Here's how the part is built. I have some questions about the finished solid (model axes, mm). A direction names the side the tool comes from. Give positions to 0.01 mm unless a question says otherwise; leave off trailing zeros. Write each loop counter-clockwise with the first axis right and the second up, starting at its lowest first coordinate (ties: lowest second). Pieces come first, ordered by that corner, then holes. Notation, with made-up numbers: (47, -31) - (54, -31) arc R22 cw to (54, -6) - close; hole circle Ø3 at (42.5, 2.5). An arc over 180 degrees is marked (long way). Use a Markdown table: item, result.
```python
from build123d import *

# Parameters (mm, degrees)
BOSS_EXTRUDE1_DEPTH      = 25.4
BOSS_EXTRUDE1_DEPTH_BACK = 25.4
SKETCH3_R                = 8.382
CUT_EXTRUDE9_DEPTH       = 95.36535858
CUT_EXTRUDE14_DEPTH      = 63.5
SKETCH14_W               = 38.1
SKETCH14_H               = 46.622003784
CUT_EXTRUDE23_DEPTH      = 12.7
CUT_EXTRUDE23_DRAFT      = -8
SKETCH13_W               = 5.08
SKETCH13_H               = 2.54
CUT_EXTRUDE22_DEPTH      = 105.116765701
FILLET4_R                = 25.4
CUT_EXTRUDE24_REACH      = 96.365
SKETCH17_R               = 7.62
SKETCH17_R_2             = 2.032
CUT_EXTRUDE25_DEPTH      = 95.36535858
FILLET5_R                = 1.27
SKETCH17_7_R             = 2.032
CUT_EXTRUDE26_DEPTH      = 12.7
SKETCH18_R               = 7.62
CUT_EXTRUDE27_DEPTH      = 12.7


with BuildPart() as part:
    # Sketch1 → Boss-Extrude1 (new, two sides: drawn at the far end of the back side and taken through both)
    with BuildSketch(Plane(origin=(0, 0, 0), x_dir=(0, 0, -1), z_dir=(1, 0, 0)).offset(-BOSS_EXTRUDE1_DEPTH_BACK)):
        Polygon((0, 0), (6.960987543, 49.53), (76.2, 49.53), (76.2, 0), align=None)
    extrude(amount=BOSS_EXTRUDE1_DEPTH + BOSS_EXTRUDE1_DEPTH_BACK)

    # Sketch3 → Cut-Extrude9 (cut, through all)
    with BuildSketch(Plane.XZ):
        with Locations(Location((0, -63.246, 0), (0, 0, 270))):
            Circle(SKETCH3_R)
        with Locations(Location((0, -25.4, 0), (0, 0, 270))):
            Circle(SKETCH3_R)
    extrude(amount=-CUT_EXTRUDE9_DEPTH, mode=Mode.SUBTRACT)

    # Sketch9 → Cut-Extrude14 (cut)
    with BuildSketch(Plane(origin=(0, 0, -76.2), x_dir=(-1, 0, 0), z_dir=(0, 0, -1))):
        Polygon((-15.24, 49.53), (-15.24, 29.21), (-11.43, 29.21), (-11.43, 25.4), (-19.05, 25.4), (-19.05, 0), (19.05, 0), (19.05, 25.4), (11.43, 25.4), (11.43, 29.21), (15.24, 29.21), (15.24, 49.53), align=None)
    extrude(amount=-CUT_EXTRUDE14_DEPTH, mode=Mode.SUBTRACT)


with BuildPart() as cut_extrude23_tool:
    # Sketch14 → Cut-Extrude23 (with draft: the straight prism first)
    with BuildSketch(Plane.XZ):
        with Locations((0, -29.661001892)):
            Rectangle(SKETCH14_W, SKETCH14_H)
    extrude(amount=-CUT_EXTRUDE23_DEPTH)
    # Cut-Extrude23: the draft: its side faces are tilted about the plane it starts from
    cut_extrude23_sides = [cut_extrude23_tool.faces().sort_by_distance(p)[0] for p in [
        (0, 6.35, -6.35),
        (-19.05, 6.35, -29.661001892),
        (0, 6.35, -52.972003784),
        (19.05, 6.35, -29.661001892),
    ]]
    draft(cut_extrude23_sides, Plane.XZ, CUT_EXTRUDE23_DRAFT)


with BuildPart() as part_1:
    add(part.part)

    # Cut-Extrude23: cut by cut_extrude23_tool
    add(cut_extrude23_tool.part, mode=Mode.SUBTRACT)

    # Sketch13 → Cut-Extrude22 (cut, through all)
    with BuildSketch(Plane.ZY.offset(25.4)):
        with Locations((-70.485, 25.4)):
            Rectangle(SKETCH13_W, SKETCH13_H)
        with Locations((-34.900987543, 25.4)):
            Rectangle(SKETCH13_W, SKETCH13_H)
    extrude(amount=-CUT_EXTRUDE22_DEPTH, mode=Mode.SUBTRACT)

    # Fillet4
    # the kernel refuses this fillet: 25.4 mm, written as the material it takes off along each edge
    with BuildSketch(Plane(origin=(-25.4, 49.53, 56.539012457), x_dir=(1, 0, 0), z_dir=(0, 0, -1)), Plane(origin=(25.4, 49.53, 56.539012457), x_dir=(0, -1, 0), z_dir=(0, 0, -1))) as fillet4_piece_1:
        with BuildLine():
            CenterArc((FILLET4_R, FILLET4_R), FILLET4_R, 180, 90)
            Line((0, FILLET4_R), (0, 0))
            Line((0, 0), (FILLET4_R, 0))
        make_face()
    extrude(amount=196.239012457, mode=Mode.SUBTRACT)

    # Cut-Extrude24: up to this face of the body (flat: up to its plane)
    cut_extrude24_end = Plane(part_1.part.faces().sort_by_distance((0, 6.245967005, -7.227813416))[0])
    # Sketch9<4> → Cut-Extrude24 (cut, up to the picked face)
    with BuildSketch(Plane(origin=(0, 0, -76.2), x_dir=(-1, 0, 0), z_dir=(0, 0, -1)), mode=Mode.PRIVATE) as cut_extrude24_sk1:
        Polygon((-15.24, 49.53), (-15.24, 29.21), (-11.43, 29.21), (-11.43, 25.4), (-19.05, 25.4), (-19.05, 0), (19.05, 0), (19.05, 25.4), (11.43, 25.4), (11.43, 29.21), (15.24, 29.21), (15.24, 49.53), align=None)
    cut_extrude24_tool1 = split(extrude(cut_extrude24_sk1.sketch, amount=-CUT_EXTRUDE24_REACH, mode=Mode.PRIVATE), bisect_by=cut_extrude24_end, keep=Keep.BOTH, mode=Mode.PRIVATE)
    add(cut_extrude24_tool1.solids().sort_by(Axis((0, 23.326156, -76.2), (0, 0, 1)))[0], mode=Mode.SUBTRACT)

    # Sketch17 → Cut-Extrude25 (cut, through all)
    with BuildSketch(Plane(origin=(0, 0, 0), x_dir=(1, 0, 0), z_dir=(0, 0.13917310096006918, 0.9902680687415698))):
        with Locations(Location((0, 23.876, 0), (0, 0, 270))):
            Circle(SKETCH17_R)
        with Locations(Location((10.524860174, 13.351139826, 0), (0, 0, 270))):
            Circle(SKETCH17_R_2)
        with Locations(Location((-10.524860174, 13.351139826, 0), (0, 0, 270))):
            Circle(SKETCH17_R_2)
    extrude(amount=-CUT_EXTRUDE25_DEPTH, mode=Mode.SUBTRACT)

    # Fillet5
    fillet5_edges = [part_1.edges().sort_by_distance(p)[0] for p in [
        (25.272680903, 26.67, -70.485),
        (-25.272680903, 26.67, -70.485),
        (25.272680903, 26.67, -34.900987543),
        (-25.272680903, 26.67, -34.900987543),
    ]]
    fillet(fillet5_edges, radius=FILLET5_R)

    # Sketch17<7> → Cut-Extrude26 (cut)
    with BuildSketch(Plane(origin=(0, 0, 0), x_dir=(1, 0, 0), z_dir=(0, 0.13917310096006918, 0.9902680687415698))):
        with Locations(Location((10.524860174, 34.400860174, 0), (0, 0, 270))):
            Circle(SKETCH17_7_R)
        with Locations(Location((-10.524860174, 34.400860174, 0), (0, 0, 270))):
            Circle(SKETCH17_7_R)
    extrude(amount=-CUT_EXTRUDE26_DEPTH, mode=Mode.SUBTRACT)

    # Sketch18 → Cut-Extrude27 (cut)
    with BuildSketch(Plane(origin=(25.4, 0, 0), x_dir=(0, 0, -1), z_dir=(1, 0, 0))):
        with Locations((22.304564874, 12.7)):
            Circle(SKETCH18_R)
    extrude(amount=-CUT_EXTRUDE27_DEPTH, mode=Mode.SUBTRACT)


solid = part_1.part
```
Item 1: Will these pins go through, and if not, where does the flat tip stop? pin 1 Ø1.5 at (x, z) = (16, -30.5) entering from -Y; pin 2 Ø8 at (y, z) = (44, -48.5) entering from -X; pin 3 Ø6 at (x, y) = (-7, 22) entering from -Z; pin 4 Ø2.5 at (x, z) = (-18.5, -34) entering from -Y.
Values:
| item | result |
|---|---|
| pin 1 | stops at y = 25.4 |
| pin 2 | stops at x = -19.83 |
| pin 3 | stops at z = -9.86 |
| pin 4 | stops at y = 0 |
Item 2: Thinking about a two-plate mould opening in X: for faces 6 (the flat face through (-11.43, 27, -44)), 7 (the flat face through (-25.4, 12, -39)), 8 (the flat face through (-20, 26, -32.361)), which applies, +X half, -X half, draft (parallel to the pull), parting line (faces both ways), or undercut?
Values:
| item | result |
|---|---|
| face 6 | undercut |
| face 7 | -X half |
| face 8 | draft |
Item 3: If we section it at B-B, the plane x = 2: Write out the boundary of the cut face in (y, z).
Values:
| item | result |
|---|---|
| outline | (0, -6.35) - (15.49, -8.53) - (16.36, -2.3) - (0, 0) - close; (30.05, -10.57) - (45.18, -12.7) - (49.45, -12.7) - (49.45, -6.95) - (30.92, -4.35) - close |
Item 4: If we section it at A-A, the plane z = -55: Write out the boundary of the cut face in (x, y), plus the area to 3 significant figures.
Values:
| item | result |
|---|---|
| outline | (-25.4, 0) - (-19.05, 0) - (-19.05, 25.4) - (-11.43, 25.4) - (-11.43, 29.21) - (-15.24, 29.21) - (-15.24, 44.45) arc R25.4 ccw to (-25.4, 24.13) - close; (11.43, 25.4) - (19.05, 25.4) - (19.05, 0) - (25.4, 0) - (25.4, 24.13) arc R25.4 ccw to (15.24, 44.45) - (15.24, 29.21) - (11.43, 29.21) - close |
| area | 614 mm2 |
Item 5: I need wall thicknesses on line 1 along X through (y, z) = (25, -12); line 2 along X through (y, z) = (13.5, -70); line 3 along Y through (x, z) = (-14.5, -59). Which ranges of each line are inside material? Lowest first, please. Write a range as [from, to].
Values:
| item | result |
|---|---|
| line 1 | x = [-25.39, -19.05], [19.05, 25.39] |
| line 2 | x = [-25.4, -19.05], [19.05, 25.4] |
| line 3 | y = [25.4, 29.21] |
Item 6: If we section it at D-D, the plane y = 42.5: Write out the boundary of the cut face in (x, z).
Values:
| item | result |
|---|---|
| outline | (-17.54, -76.2) - (-15.24, -76.2) - (-15.24, -12.32) - (15.24, -12.32) - (15.24, -76.2) - (17.54, -76.2) - (17.54, -5.97) - (-17.54, -5.97) - close |
Item 7: For faces 1 (the flat face through (-20, 23, -76.2)), 2 (the cylindrical face through (2.289, 16.015, -5.381)), 3 (the flat face through (22, 24.13, -71)), 4 (the flat face through (15, 25.4, -53)), 5 (the cylindrical face through (22.269, 20.255, -21.313)), which set-ups out of +Z, -Z, +X, -X, +Y, -Y let a thin tool reach every point of the face, with its end or its side?
Values:
| item | result |
|---|---|
| face 1 | -Z, +X, -X, +Y, -Y |
| face 2 | none |
| face 3 | +X, -X |
| face 4 | -Z, -Y |
| face 5 | +X |
Item 8: If we section it at C-C, the plane y = 9: Write out the boundary of the cut face in (x, z), plus the area to 3 significant figures.
Values:
| item | result |
|---|---|
| outline | (-25.4, -76.2) - (-19.05, -76.2) - (-19.05, -7.61) - (19.05, -7.61) - (19.05, -15.64) - (25.4, -15.64) - (25.4, -1.26) - (-25.4, -1.26) - close; (19.05, -76.2) - (25.4, -76.2) - (25.4, -28.97) - (19.05, -28.97) - close |
| area | 1,110 mm2 |
